Can you work these out from the model? Positions are in its coordinate system, mm. Face numbers are marked on the shaded views. Give positions to 0.01 mm unless a question says otherwise; leave off trailing zeros. Write each loop counter-clockwise with the first axis right and the second up, starting at its lowest first coordinate (ties: lowest second). Pieces come first, ordered by that corner, then holes. Notation, with made-up numbers: M -32.5,45 L 3.5,45 A18 ccw 3.5,56 Z; hole C 71.5,76 d11. An arc over 180 degrees is marked long. Write each question's results on one line, items separated by ' | '.
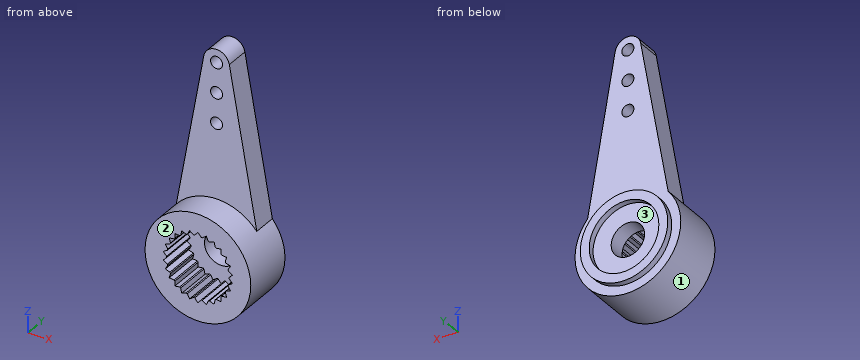
from build123d import *

# Parameters (mm, degrees)
SKETCH1_R               = 4.4
BOSS_EXTRUDE1_DEPTH     = 4.4
BOSS_EXTRUDE2_DEPTH     = 2
SKETCH3_R               = 3.64
SKETCH3_R_2             = 2.9
BOSS_EXTRUDE3_DEPTH     = 0.5
SKETCH4_R               = 1.39
CUT_EXTRUDE1_DEPTH      = 5.4
SKETCH5_R               = 0.5
CUT_EXTRUDE2_DEPTH      = 5.9
LPATTERN1_COUNT         = 3
LPATTERN1_PITCH         = 2.5
MIRROR1_COPY_1_SKETCH_R = 0.5
MIRROR1_COPY_1_DEPTH    = 5.9
MIRROR1_COPY_2_SKETCH_R = 0.5
MIRROR1_COPY_2_DEPTH    = 5.9
CUT_EXTRUDE4_DEPTH      = 3
CIRPATTERN2_COUNT       = 26
SKETCH9_R               = 2.6
CUT_EXTRUDE5_DEPTH      = 3
CUT_EXTRUDE6_DEPTH      = 4.9


with BuildPart() as part:
    # Sketch1 → Boss-Extrude1 (new body)
    with BuildSketch(Plane(origin=(0, 0, 0), x_dir=(1, 0, 0), z_dir=(0, 1, 0))):
        Circle(SKETCH1_R)
    extrude(amount=BOSS_EXTRUDE1_DEPTH)

    # Sketch2 → Boss-Extrude2 (add)
    with BuildSketch(Plane(origin=(0, 4.4, 0), x_dir=(1, 0, 0), z_dir=(0, 1, 0))):
        with BuildLine():
            Line((-1.063592373, 15.807540032), (-3.347342764, 2.855747962))
            ThreePointArc((-3.347342764, 2.855747962), (0, 4.4), (3.347342764, 2.855747962))
            Line((3.347342764, 2.855747962), (1.063592373, 15.807540032))
            ThreePointArc((1.063592373, 15.807540032), (0, 16.7), (-1.063592373, 15.807540032))
        make_face()
    boss_extrude2 = extrude(amount=-BOSS_EXTRUDE2_DEPTH)

    # Sketch3 → Boss-Extrude3 (add)
    with BuildSketch(Plane(origin=(0, 4.4, 0), x_dir=(-1, 0, 0), z_dir=(0, -1, 0))):
        Circle(SKETCH3_R)
        Circle(SKETCH3_R_2, mode=Mode.SUBTRACT)
    extrude(amount=-BOSS_EXTRUDE3_DEPTH)

    # Sketch4 → Cut-Extrude1 (cut, through all)
    with BuildSketch(Plane(origin=(0, 4.4, 0), x_dir=(-1, 0, 0), z_dir=(0, -1, 0))):
        Circle(SKETCH4_R)
    extrude(amount=CUT_EXTRUDE1_DEPTH, mode=Mode.SUBTRACT)

    # Sketch5 → Cut-Extrude2 (cut, through all)
    with BuildSketch(Plane(origin=(0, 0, 0), x_dir=(-1, 0, 0), z_dir=(0, -1, 0))):
        with Locations((0, 15.62)):
            Circle(SKETCH5_R)
    cut_extrude2 = extrude(amount=-CUT_EXTRUDE2_DEPTH, mode=Mode.SUBTRACT)

    # LPattern1: Cut-Extrude2 ×3
    with Locations(*[(0, 0, i * LPATTERN1_PITCH) for i in range(1, LPATTERN1_COUNT)]):
        add(cut_extrude2, mode=Mode.SUBTRACT)

    # Mirror1: Boss-Extrude2, Cut-Extrude2 across plane
    add(boss_extrude2.mirror(Plane.XY))
    add(cut_extrude2.mirror(Plane.XY), mode=Mode.SUBTRACT)

    # Mirror1 copy 1 sketch → Mirror1 copy 1 (cut, through all)
    with BuildSketch(Plane(origin=(0, 0, -2.5), x_dir=(-1, 0, 0), z_dir=(0, -1, 0))):
        with Locations((0, -15.62)):
            Circle(MIRROR1_COPY_1_SKETCH_R)
    extrude(amount=-MIRROR1_COPY_1_DEPTH, mode=Mode.SUBTRACT)

    # Mirror1 copy 2 sketch → Mirror1 copy 2 (cut, through all)
    with BuildSketch(Plane(origin=(0, 0, -5), x_dir=(-1, 0, 0), z_dir=(0, -1, 0))):
        with Locations((0, -15.62)):
            Circle(MIRROR1_COPY_2_SKETCH_R)
    extrude(amount=-MIRROR1_COPY_2_DEPTH, mode=Mode.SUBTRACT)

    # Sketch8 → Cut-Extrude4 (cut)
    with BuildSketch(Plane(origin=(0, 0, 0), x_dir=(-1, 0, 0), z_dir=(0, -1, 0))):
        with BuildLine():
            Line((0, -2.9), (0.262912611, -2.586672952))
            ThreePointArc((0.262912611, -2.586672952), (0, -2.6), (-0.262912611, -2.586672952))
            Line((-0.262912611, -2.586672952), (0, -2.9))
        make_face()
    cut_extrude4 = extrude(amount=-CUT_EXTRUDE4_DEPTH, mode=Mode.SUBTRACT)

    # CirPattern2: Cut-Extrude4 ×26 about axis
    cirpattern2_axis = Axis((0, 0, 0), (0, 1, 0))
    for i in range(1, CIRPATTERN2_COUNT):
        add(cut_extrude4.rotate(cirpattern2_axis, i * 360 / CIRPATTERN2_COUNT), mode=Mode.SUBTRACT)

    # Sketch9 → Cut-Extrude5 (cut)
    with BuildSketch(Plane(origin=(0, 0, 0), x_dir=(-1, 0, 0), z_dir=(0, -1, 0))):
        Circle(SKETCH9_R)
    extrude(amount=-CUT_EXTRUDE5_DEPTH, mode=Mode.SUBTRACT)

    # Horn Trim Sketch → Cut-Extrude6 (cut)
    with BuildSketch(Plane.XZ):
        with BuildLine():
            Line((-4.4, 0), (-4.4, -16.7))
            Line((-4.4, -16.7), (4.4, -16.7))
            Line((4.4, -16.7), (4.4, 0))
            ThreePointArc((4.4, 0), (0, -4.4), (-4.4, 0))
        make_face()
    extrude(amount=-CUT_EXTRUDE6_DEPTH, mode=Mode.SUBTRACT)


solid = part.part
Item 1: If I drill on line 1 (Z direction, x = 0, y = 3.5); line 2 (Z direction, x = 0, y = 4.7); line 3 (Y direction, x = 0, z = -2.25), over which ranges is the centre line in solid material (lowest first)? Write a range as from..to.
Geometry says:
line 1: z = -4.4..-1.39, 1.39..10.12, 11.12..12.62, 13.62..15.12, 16.12..16.7 | line 2: z = -3.64..-2.9, 2.9..3.64 | line 3: y = 3..4.4
Item 2: I'm going to push flat-ended pins straight in: pin 1 (1.5 mm diameter, centred on x = -1.5, y = 2, fed in from -Z); pin 2 (1 mm diameter, centred on x = 0, z = -2, fed in from +Y); pin 3 (4.5 mm diameter, centred on x = 0, z = 0, fed in from -Y). Where does each tip first touch, or does it pass through?
Geometry says:
pin 1: stops at z = -4.34 | pin 2: stops at y = 4.4 | pin 3: stops at y = 3
Item 3: I want a section at C-C, the plane z = 10.62. Please give me the cut outline in (x, y).
Geometry says:
outline: M -1.98,2.4 L -0.5,2.4 L -0.5,4.4 L -1.98,4.4 Z; M 0.5,2.4 L 1.98,2.4 L 1.98,4.4 L 0.5,4.4 Z
Item 4: I want a section at B-B, the plane z = 15.62. Please give me the cut outline in (x, y).
Geometry says:
outline: M -1.1,2.4 L -0.5,2.4 L -0.5,4.4 L -1.1,4.4 Z; M 0.5,2.4 L 1.1,2.4 L 1.1,4.4 L 0.5,4.4 Z
Item 5: I want a section at A-A, the plane y = 4.1. Please give me the cut outline in (x, z).
Geometry says:
outline: M -3.35,2.86 A4.4 ccw long 3.35,2.86 L 1.06,15.81 A1.08 ccw -1.06,15.81 Z; hole C 0,0 d2.78; hole C 0,10.62 d1; hole C 0,13.12 d1; hole C 0,15.62 d1
Item 6: I want a section at D-D, the plane z = 7.5. Please give me the cut outline in (x, y), and give its area (3 significant figures).
Geometry says:
outline: M -2.53,2.4 L 2.53,2.4 L 2.53,4.4 L -2.53,4.4 Z | area: 10.1 mm2
Item 7: Thinking about a two-plate mould opening in X: for the marked faces 1, 2 and 3, which applies, +X half, -X half, draft (parallel to the pull), parting line (faces both ways), or undercut?
Geometry says:
face 1: parting line | face 2: draft | face 3: undercut
